For this review, use the dimensioned drawing (mm, ordinates from the lowest corner) and the shaded views. Round coordinates to 2 decimals unless told otherwise and drop trailing zeros. Write each loop counter-clockwise with the first axis right and the second up, starting at its lowest first coordinate (ties: lowest second). Pieces come first, ordered by that corner, then holes.
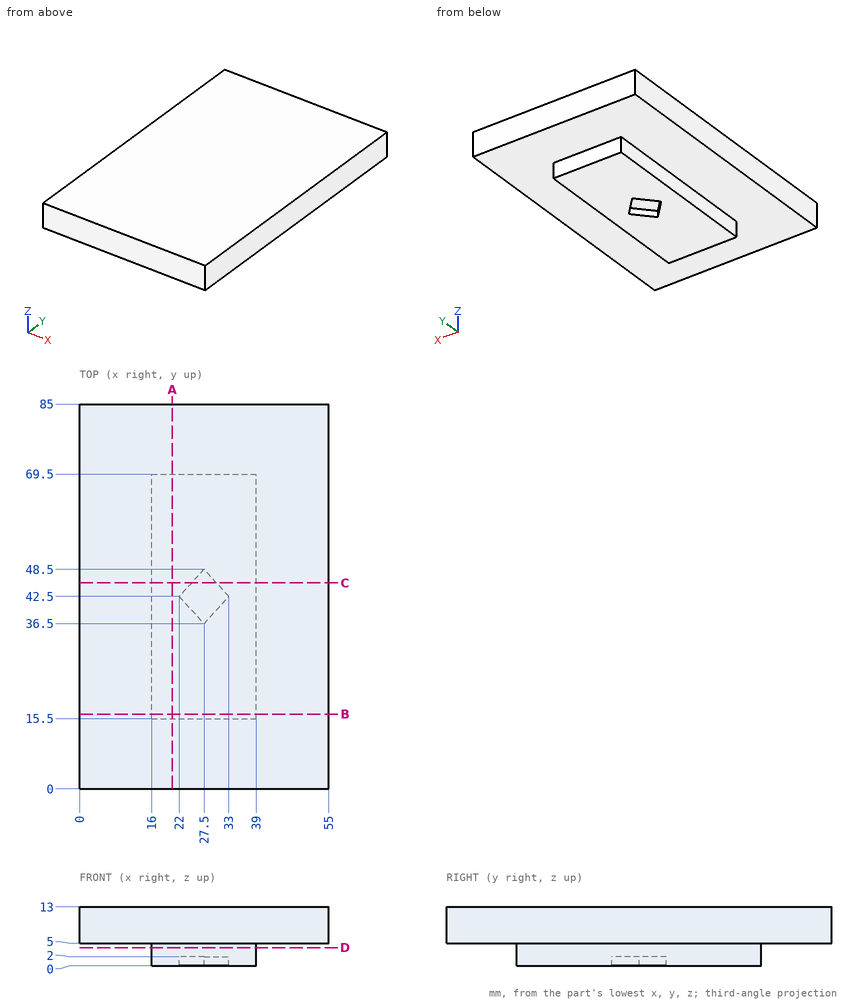
1) Add section B-B on y = 16.5. State the section outline as (x, z) points.
2) Add section C-C on y = 45.5. State the section outline as (x, z) points, and give its area (3 significant figures).
3) For line 1 along Z through (x, y) = (17.5, 8.5); line 2 along X through (y, z) = (23, 1.75); line 3 along Y through (x, z) = (21.5, 2.5), list the stretches that pass through material, from the lowest coordinate up.
4) Add section A-A on x = 20.5. State the section outline as (y, z) points, and give its area (3 significant figures).
5) For P1, Ø5.5, axis at y = 45.5, z = 2, coming from the +X side; P2, Ø3.5, axis at x = 27, y = 43.5, coming from the -Z side; P3, Ø5.5, axis at x = 26.5, z = 1.5, coming from the -Y side, all flat-tipped, find the tip position at first contact; note any pin that passes through.
6) Add section D-D on z = 4. State the section outline as (x, y) points, and give its area (3 significant figures).
Computed:
1. outline: (0, 5) - (16, 5) - (16, 0) - (39, 0) - (39, 5) - (55, 5) - (55, 13) - (0, 13) - close
2. outline: (0, 5) - (16, 5) - (16, 0) - (24.75, 0) - (24.75, 2) - (30.25, 2) - (30.25, 0) - (39, 0) - (39, 5) - (55, 5) - (55, 13) - (0, 13) - close
2. area: 544 mm2
3. line 1: z = 5 to 13
3. line 2: x = 16 to 39
3. line 3: y = 15.5 to 69.5
4. outline: (0, 5) - (15.5, 5) - (15.5, 0) - (69.5, 0) - (69.5, 5) - (85, 5) - (85, 13) - (0, 13) - close
4. area: 950 mm2
5. P1: stops at x = 39
5. P2: stops at z = 2
5. P3: stops at y = 15.5
6. outline: (16, 15.5) - (39, 15.5) - (39, 69.5) - (16, 69.5) - close
6. area: 1,240 mm2
